from build123d import *

# Parameters (mm, degrees)
FILETE2_R     = 7
FILETE3_R     = 5
CHANFRO1_SIZE = 3
FILETE6_R     = 1


with BuildPart() as part:
    # Esboço1 → Revolução1 (revolve)
    with BuildSketch(Plane(origin=(0, 0, 0), x_dir=(1, 0, 0), z_dir=(0, 1, 0)), mode=Mode.PRIVATE) as revolu_o1_sk:
        Polygon((0.000828852, 3.2), (66, 3.2), (66, 6.5), (61.2, 6.5), (61.2, 5), (56.2, 5), (56.2, 6.4), (16.000828852, 6.4), (12.000828852, 5.2), (4.000828852, 5.2), (0.000828852, 4), align=None)
    revolve(revolu_o1_sk.sketch.rotate(Axis((0, 0, 0), (1, 0, 0)), 180), axis=Axis((0, 0, 0), (1, 0, 0)))

    # Filete2
    filete2_edges = [part.edges().sort_by_distance(p)[0] for p in [
        (4.000828852, 0, -5.2),
    ]]
    fillet(filete2_edges, radius=FILETE2_R)

    # Filete3
    filete3_edges = [part.edges().sort_by_distance(p)[0] for p in [
        (12.000828852, 0, -5.2),
    ]]
    fillet(filete3_edges, radius=FILETE3_R)

    # Chanfro1
    chanfro1_edges = [part.edges().sort_by_distance(p)[0] for p in [
        (66, 0, -3.2),
    ]]
    chamfer(chanfro1_edges, length=CHANFRO1_SIZE)

    # Filete6
    filete6_edges = [part.edges().sort_by_distance(p)[0] for p in [
        (0.000828852, 0, -4),
    ]]
    fillet(filete6_edges, radius=FILETE6_R)


solid = part.part
Could you check a few things on this model? Use its own coordinates, in mm. A direction names the side the tool comes from. Coordinates: 2 decimals unless noted, no trailing zeros. Order: outer loops, then holes, each group sorted by start corner. A loop starts at its lowest first (then second) coordinate and runs counter-clockwise, first axis right, second up. Notation, with made-up numbers: (3.5, 30) - (36.5, 30) arc R28 cw to (36.5, 63) - close; hole circle Ø3 at (58, 17). An arc over 180 degrees is marked (long way). Answer in a Markdown table with one row per item. Add a question column.
(1) I need wall thicknesses on L1, parallel to Y at x = 28.5, z = 0; L2, parallel to Z at x = 4.5, y = 0.25; L3, parallel to Z at x = 50, y = -1.25. Which ranges of each line are inside material? Lowest first, please.
(2) On a 3-axis mill with a long thin cutter (end or side, diameter ignored), from which of +Z, -Z, +X, -X, +Y, -Y can I reach the whole of each face in a straight line? I mean faces 1 (the face through (35.819, -1.922, 6.104)), 2 (the face through (56.2, 2, 5)), 3 (the face through (63.19, 3.31, -0.73)). Say none if no direction works.
(3) Will these pins go through, and if not, where does the flat tip stop? pin 1 (3 mm diameter, centred on x = 16.5, y = -4, fed in from -Z); pin 2 (1 mm diameter, centred on x = 59, y = -1.5, fed in from -Z); pin 3 (4 mm diameter, centred on x = 51, z = 4.5, fed in from +Y); pin 4 (4 mm diameter, centred on y = 0, z = 0, fed in from -X).
(4) If we section it at A-A, the plane x = 25.5: Please give me the cut outline in (y, z), then the cut area to 3 significant figures.
(5) If we mould it in two halves opening along Y, with no side actions, what happens to faces 4 (the face through (61.2, 5, 2)), 5 (the face through (63.566, 3.955, -5.158)), 6 (the face through (31.941, -0.961, 3.052))? For each: released by +Y, released by -Y, zero draft, split by the parting line, or undercut.
Results are:
| question | item | result |
|---|---|---|
| 1 | L1 | y = -6.4 to -3.2, 3.2 to 6.4 |
| 1 | L2 | z = -5.17 to -3.19, 3.19 to 5.17 |
| 1 | L3 | z = -6.28 to -2.95, 2.95 to 6.28 |
| 2 | face 1 | -X |
| 2 | face 2 | none |
| 2 | face 3 | +X |
| 3 | pin 1 | stops at z = -5.89 |
| 3 | pin 2 | stops at z = -4.9 |
| 3 | pin 3 | stops at y = 5.89 |
| 3 | pin 4 | passes through |
| 4 | outline | circle Ø12.8 at (0, 0); hole circle Ø6.4 at (0, 0) |
| 4 | area | 96.5 mm2 |
| 5 | face 4 | zero draft |
| 5 | face 5 | split by the parting line |
| 5 | face 6 | undercut |
